```python
from build123d import *

# Parameters (mm, degrees)
F2_R      = 33.0835
F3_R      = 5.461
F5_T      = -2.54
F8_DEPTH  = 90.424
F10_DEPTH = 2.286
F11_R     = 26.7767955421
F12_DEPTH = 20.574


with BuildPart() as f4:
    # F2 (on offset) → F4 section 0
    with BuildSketch(Plane.XY.offset(87.376)):
        Circle(F2_R)
    # F3 (on offset) → F4 section 1
    with BuildSketch(Plane.XY.offset(-80.264)):
        Circle(F3_R)
    loft()

    # F5
    f5_openings = [f4.faces().sort_by_distance(p)[0] for p in [
        (0, 0, 87.376),
    ]]
    offset(amount=F5_T, openings=f5_openings, kind=Kind.INTERSECTION)

    # F7 (on offset) → F8 (cut)
    with BuildSketch(Plane.XZ.offset(-33.274)):
        Polygon((7.2469562292, -55.821005255), (-10.5406511575, -47.1849963069), (-7.9627372324, -54.7898411751), (5.8291028254, -61.6213157773), align=None)
        Polygon((-12.987045992, -28.3675191), (-10.5406511575, -35.5843827128), (6.2097211414, -43.0105263684), (8.6648091674, -36.3577567041), align=None)
        Polygon((-16.3409579545, -4.6494142152), (-13.8919390738, -15.9922353923), (4.0245633572, -20.6324812025), (11.5005131811, -11.3519905135), align=None)
        Polygon((-19.2826890827, 16.0057449445), (-16.3409579545, 7.3276394978), (8.6648091674, 0), (15.4022630304, 6.0269851238), align=None)
        Polygon((-19.2826890827, 39.1713567078), (-19.2826890827, 29.1993264109), (3.5543837585, 22.1851039678), (11.5005131811, 27.8113555213), align=None)
    extrude(amount=F8_DEPTH, mode=Mode.SUBTRACT)

    # F9 (on offset) → F10 (join)
    with BuildSketch(Plane.XY.offset(87.376)):
        with BuildLine():
            ThreePointArc((-35.9650850296, -12.119741179), (-38.0913082045, -20.5690913054), (-29.6588800848, -22.761464119))
            ThreePointArc((-29.6588800848, -22.761464119), (-4.2577579723, -37.2069935895), (24.5350878686, -32.2207771242))
            ThreePointArc((24.5350878686, -32.2207771242), (33.7905432246, -32.7064272786), (36.1621566117, -23.7468089908))
            ThreePointArc((36.1621566117, -23.7468089908), (41.1105620393, -0.3473779509), (32.0237055421, 21.7761192471))
            ThreePointArc((32.0237055421, 21.7761192471), (31.6611388158, 31.0655624038), (22.3673284054, 30.8412928134))
            ThreePointArc((22.3673284054, 30.8412928134), (0.3392668677, 39.5477499116), (-21.7761211097, 31.0655624038))
            ThreePointArc((-21.7761211097, 31.0655624038), (-30.1897966866, 32.5650475303), (-31.6295698285, 24.1409484297))
            ThreePointArc((-31.6295698285, 24.1409484297), (-41.9013508233, 6.9795624895), (-35.9650850296, -12.119741179))
        make_face()
    extrude(amount=F10_DEPTH)

    # F11 (on face) → F12 (cut)
    with BuildSketch(Plane.XY.offset(89.662)):
        with Locations((1.6233043279, 0)):
            Circle(F11_R)
    extrude(amount=-F12_DEPTH, mode=Mode.SUBTRACT)


solid = f4.part
```
The model under review builds one solid part; all positions refer to its coordinate system, in mm. A direction names the side the tool comes from. Give positions to 0.01 mm unless a question says otherwise; leave off trailing zeros. Loops run counter-clockwise (first coordinate to the right, second up) from the corner with the lowest first, then second, coordinate; pieces in that order, holes last. Notation, with made-up numbers: (84, 61) - (106, 61) arc R15 ccw to (106, 78) - close; hole circle Ø6 at (43, 66). An arc over 180 degrees is marked (long way). Answer as a JSON object with one key per item and string values.
Q1. For faces 1 (the flat face through (7.42, -7.99, -39.73)), 2 (the cylindrical face through (31.765, 30.966, 88.503)), 3 (the cylindrical face through (28.397, -0.427, 71.26)), 4 (the conical face through (17.702, 5.575, 14.851)), list the 3-axis set-ups (+Z, -Z, +X, -X, +Y, -Y) from which the entire face can be reached by the end or side of a thin tool; tool diameter is ignored.
Worked out:
{"face 1": "+Y, -Y", "face 2": "+Z, -Z", "face 3": "+Z", "face 4": "none"}
Q2. To check wall thickness, follow line 1 along Z through (x, y) = (-22, 28); line 2 along Y through (x, z) = (-9, 22); line 3 along Y through (x, z) = (-2, 72). State the ranges of each line that lie inside material, in increasing order.
Worked out:
{"line 1": "z = 87.38 to 89.66", "line 2": "y = -20.42 to -17.57, 17.57 to 20.42", "line 3": "y = -30.48 to -27.9, 27.9 to 30.48"}
Q3. Insertion check: pin 1 (2 mm diameter, centred on y = -1.5, z = -23, fed in from -X); pin 2 (8 mm diameter, centred on x = -4.5, z = 11, fed in from +Y); pin 3 (9 mm diameter, centred on y = -10.5, z = 33, fed in from +X). Each pin has a flat end and moves straight along its axis. Give the tip position at first contact, or say it passes through.
Worked out:
{"pin 1": "stops at x = -15.01", "pin 2": "stops at y = 20.92", "pin 3": "stops at x = 23.59"}
Q4. Add section D-D on z = 36.5. State the section outline as (x, y) points.
Worked out:
{"outline": "(-19.28, -15.44) - (-19.28, -10.85) arc R22.13 cw to (-19.28, 10.85) - (-19.28, 15.44) arc R24.7 ccw to start; (-12.04, -21.57) arc R24.7 ccw (long way) to (-12.04, 21.57) - (-12.04, 18.56) arc R22.13 cw (long way) to (-12.04, -18.56) - close"}
Q5. Add section B-B on x = 0. Count the separate pieces of the cut face and the enclosed holes in it, plus the area to 3 significant figures.
Worked out:
{"separate pieces": "11", "enclosed holes": "0", "area": "721 mm^2"}
Q6. Add section C-C on z = 71. State the section outline as (x, y) points, plus the area to 3 significant figures.
Worked out:
{"outline": "circle Ø60.77 at (0, 0); hole (18.2, -21.03) arc R26.78 ccw to (18.2, 21.03) arc R27.81 ccw (long way) to start", "area": "452 mm^2"}
Q7. Add section A-A on z = -39. State the section outline as (x, y) points, plus the area to 3 significant figures.
Worked out:
{"outline": "(-2.84, -11.93) - (-2.84, -9.26) arc R9.69 cw to (-2.84, 9.26) - (-2.84, 11.93) arc R12.26 ccw to start; (7.69, -9.55) arc R12.26 ccw to (7.69, 9.55) - (7.69, 5.89) arc R9.69 cw to (7.69, -5.89) - close", "area": "119 mm^2"}
